Input: part model. Units: mm. Frame: model coordinates. Face numbers are marked on the shaded views. A direction names the side the tool comes from. Round coordinates to 2 decimals unless told otherwise and drop trailing zeros. Order: outer loops, then holes, each group sorted by start corner. A loop starts at its lowest first (then second) coordinate and runs counter-clockwise, first axis right, second up. Notation, with made-up numbers: M -10.5,-27.75 L -6.5,-27.75 A5 cw -6.5,-20.75 Z; hole C -24,23.25 d10. An arc over 180 degrees is marked long. One line per question, with ' | ' between items.
```python
from build123d import *

# Parameters (mm, degrees)
F3_DEPTH = 1.42
F1_W     = 8.6
F1_H     = 1
F4_DEPTH = 2.5
F2_W     = 8.6
F2_H     = 3.5
F5_DEPTH = 2.2


with BuildPart() as f3:
    # F0 (on Front) → F3 (new body)
    with BuildSketch(Plane.XZ):
        Polygon((3.628443, 25.740858), (-14.121557, 25.740858), (-14.121557, 23.990858), (-13.371557, 23.990858), (-13.371557, 20.940858), (-14.121557, 20.940858), (-14.121557, 19.190858), (3.628443, 19.190858), (3.628443, 20.940858), (2.878443, 20.940858), (2.878443, 23.990858), (3.628443, 23.990858), align=None)
    extrude(amount=F3_DEPTH)

    # F1 (on face) → F4 (join)
    with BuildSketch(Plane.XZ):
        with Locations((-2.571557, 20.319503)):
            Rectangle(F1_W, F1_H)
    extrude(amount=F4_DEPTH)

    # F2 (on face) → F5 (join)
    with BuildSketch(Plane.XZ):
        with Locations((-2.571557, 23.990858)):
            Rectangle(F2_W, F2_H)
    extrude(amount=F5_DEPTH)


solid = f3.part
```
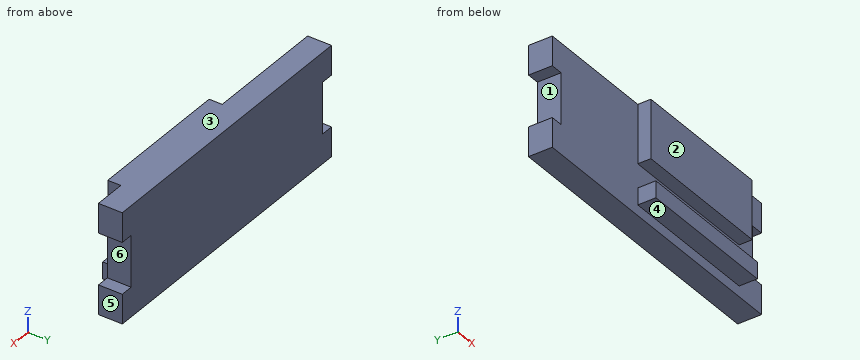
Item 1: Section query A-A, the plane z = 20.5. Return loops of the section in (x, y).
Report:
outline: M -14.12,-1.42 L -6.87,-1.42 L -6.87,-2.5 L 1.73,-2.5 L 1.73,-1.42 L 3.63,-1.42 L 3.63,0 L -14.12,0 Z
Item 2: Mould query, pull axis Z, two halves, no side actions, for the marked faces 1, 2 and 3. Classes: +Z half, -Z half, draft (parallel to the pull), parting line (faces both ways), or undercut.
Report:
face 1: undercut | face 2: draft | face 3: +Z half
Item 3: Section query C-C, the plane y = -0.25. Return loops of the section in (x, z).
Report:
outline: M -14.12,19.19 L 3.63,19.19 L 3.63,20.94 L 2.88,20.94 L 2.88,23.99 L 3.63,23.99 L 3.63,25.74 L -14.12,25.74 L -14.12,23.99 L -13.37,23.99 L -13.37,20.94 L -14.12,20.94 Z
Item 4: First-contact query: pin 1 (0.9 mm diameter, centred on y = -2, z = 23.5, fed in from -X); pin 2 (1 mm diameter, centred on x = 1.5, z = 24.5, fed in from -Y); pin 3 (1 mm diameter, centred on x = -7, z = 20, fed in from -Y); pin 4 (0.9 mm diameter, centred on x = -1, y = -2, fed in from -Z). Flat tips, straight axial feed; report the tip coordinate or a pass-through.
Report:
pin 1: x = -6.87 | pin 2: y = -2.2 | pin 3: y = -2.5 | pin 4: z = 19.82
Item 5: Section query B-B, the plane x = -4.25. Return loops of the section in (y, z), plus the area to 3 significant figures.
Report:
outline: M -2.5,19.82 L -1.42,19.82 L -1.42,19.19 L 0,19.19 L 0,25.74 L -2.2,25.74 L -2.2,22.24 L -1.42,22.24 L -1.42,20.82 L -2.5,20.82 Z | area: 13.1 mm²
Item 6: Access query for the marked faces 4, 5 and 6. Directions: +Z, -Z, +X, -X, +Y, -Y. A direction counts if a zero-diameter tool reaches every point of the face in a straight line with its end or side. Return the directions, or none.
Report:
face 4: -Z, +X, -X, -Y | face 5: +Z, -Z, +X, +Y, -Y | face 6: +X, +Y, -Y
Item 7: Line query: line 1 along X through (y, z) = (-0.1, 23); line 2 along X through (y, z) = (-2.15, 24.25); line 3 along Y through (x, z) = (0, 24.25). Output: solid intervals per line, ascending. Write a range as from..to.
Report:
line 1: -13.37..2.88 | line 2: -6.87..1.73 | line 3: -2.2..0
Item 8: Section query D-D, the plane z = 25. Return loops of the section in (x, y), plus the area to 3 significant figures.
Report:
outline: M -14.12,-1.42 L -6.87,-1.42 L -6.87,-2.2 L 1.73,-2.2 L 1.73,-1.42 L 3.63,-1.42 L 3.63,0 L -14.12,0 Z | area: 31.9 mm²
